Design review of the part built by this model. Coordinates are the model's own, in mm. Give positions to 0.01 mm unless a question says otherwise; leave off trailing zeros. Loops run counter-clockwise (first coordinate to the right, second up) from the corner with the lowest first, then second, coordinate; pieces in that order, holes last. Notation, with made-up numbers: (14, 15) -> (26, 15) arc R6 cw to (26, 22) -> close; hole circle Ø9 at (-1.5, 23). An arc over 180 degrees is marked (long way). Answer as CSV lines item,"result".
Autodesk Inventor part; units mm, degrees
ref_plane "YZ Plane" through (0, 0, 0) normal (1, 0, 0) x (0, 1, 0)
ref_plane "XZ Plane" through (0, 0, 0) normal (0, 1, 0) x (-1, 0, 0)
ref_plane "XY Plane" through (0, 0, 0) normal (0, 0, 1) x (1, 0, 0)
sketch "Szkic1" plane through (0, 0, 0) normal (0, 0, 1) x (1, 0, 0)
  line L0 (0, 0) -> (40, 0) construction
  line L1 (0, -10) -> (40, -10)
  line L2 (40, 10) -> (0, 10)
  arc A0 (0, 10) -> (0, -10) centre (0, 0) ccw
  arc A1 (40, -10) -> (40, 10) centre (40, 0) ccw
  point P0 (20, 0)
  dimension "d0" = 40
  dimension "d1" = 20
extrude "Wyciągnięcie proste1" add sketch "Szkic1" along normal blind 3
hole "Otwór1" at (0, 0, 0) at (40, 0, 0) direction (0, 0, 1) diameter 8 end through all
properties part number "ramie_2_wahacza"
Q1. The part is to be moulded in two halves that separate along Y. For faces 1 (the flat face through (20, -10, 1)), 2 (the cylindrical face through (36.034, -0.521, 1.521)), 3 (the flat face through (20, 10, 1)), say which applies: pulls with the +Y half, pulls with the -Y half, needs draft (parallel to the pull), parting line crosses it, or undercut.
Filled sheet:
face 1,"pulls with the -Y half"
face 2,"undercut"
face 3,"pulls with the +Y half"
Q2. We need section D-D, the plane y = 2.75. State the section outline as (x, z) points, and give its area (3 significant figures).
Filled sheet:
outline,"(-9.61, 0) -> (-2.9, 0) -> (-2.9, 3) -> (-9.61, 3) -> close; (2.9, 0) -> (37.1, 0) -> (37.1, 3) -> (2.9, 3) -> close; (42.9, 0) -> (49.61, 0) -> (49.61, 3) -> (42.9, 3) -> close"
area,"143 mm^2"
Q3. To check wall thickness, follow probe 1 along X at (y, z) = (0, 1.05); probe 2 along Y at (x, z) = (0, 0.95); probe 3 along X at (y, z) = (3.5, 1.7). State the ranges of each line that lie inside material, in increasing order. Write a range as from..to.
Filled sheet:
probe 1,"x = -10..-4, 4..36, 44..50"
probe 2,"y = -10..-4, 4..10"
probe 3,"x = -9.37..-1.94, 1.94..38.06, 41.94..49.37"
Q4. We need section B-B, the plane z = 0.5. State the section outline as (x, y) points.
Filled sheet:
outline,"(0, -10) -> (40, -10) arc R10 ccw to (40, 10) -> (0, 10) arc R10 ccw to start; hole circle Ø8 at (0, 0); hole circle Ø8 at (40, 0)"
Q5. We need section C-C, the plane x = -2.5. State the section outline as (y, z) points.
Filled sheet:
outline,"(-9.68, 0) -> (-3.12, 0) -> (-3.12, 3) -> (-9.68, 3) -> close; (3.12, 0) -> (9.68, 0) -> (9.68, 3) -> (3.12, 3) -> close"
Q6. We need section A-A, the plane y = 0. State the section outline as (x, z) points, and give its area (3 significant figures).
Filled sheet:
outline,"(-10, 0) -> (-4, 0) -> (-4, 3) -> (-10, 3) -> close; (4, 0) -> (36, 0) -> (36, 3) -> (4, 3) -> close; (44, 0) -> (50, 0) -> (50, 3) -> (44, 3) -> close"
area,"132 mm^2"
Q7. Clearance check with flat-ended pins moving along their axes: pin 1 Ø1.5 at (y, z) = (-2.5, 2.5) entering from -X; pin 2 Ø1 at (y, z) = (-5, 2) entering from -X; pin 3 Ø12 at (x, y) = (32, 6) entering from -Z. State where each tip first meets the part, or that it passes through.
Filled sheet:
pin 1,"stops at x = -9.85"
pin 2,"stops at x = -8.93"
pin 3,"stops at z = 0"
